Can you work these out from the model? Positions are in its coordinate system, mm. A direction names the side the tool comes from. Give positions to 0.01 mm unless a question says otherwise; leave off trailing zeros. Loops run counter-clockwise (first coordinate to the right, second up) from the corner with the lowest first, then second, coordinate; pieces in that order, holes last.
from build123d import *

# Parameters (mm, degrees)
SKETCH1_R           = 4
BOSS_EXTRUDE1_DEPTH = 5
CUT_EXTRUDE1_DEPTH  = 5


with BuildPart() as part:
    # Sketch1 → Boss-Extrude1 (new body)
    with BuildSketch(Plane.XY):
        with BuildLine():
            Line((-15, 6.5), (15, 6.5))
            ThreePointArc((15, 6.5), (21.5, 0), (15, -6.5))
            Line((15, -6.5), (-15, -6.5))
            ThreePointArc((-15, -6.5), (-21.5, 0), (-15, 6.5))
        make_face()
        with Locations((-15, 0)):
            Circle(SKETCH1_R, mode=Mode.SUBTRACT)
        with Locations((15, 0)):
            Circle(SKETCH1_R, mode=Mode.SUBTRACT)
    extrude(amount=BOSS_EXTRUDE1_DEPTH)

    # Sketch2 → Cut-Extrude1 (cut)
    with BuildSketch(Plane(origin=(21.5, 0, 0), x_dir=(0, 0, -1), z_dir=(1, 0, 0))):
        with BuildLine():
            ThreePointArc((-3.75, 0), (-2.5, -1.25), (-1.25, 0))
            Line((-1.25, 0), (-3.75, 0))
        make_face()
        with BuildLine():
            Line((-3.75, 0), (-1.25, 0))
            ThreePointArc((-1.25, 0), (-2.5, 1.25), (-3.75, 0))
        make_face()
    cut_extrude1 = extrude(amount=-CUT_EXTRUDE1_DEPTH, mode=Mode.SUBTRACT)

    # Mirror1: Cut-Extrude1 across plane
    add(cut_extrude1.mirror(Plane(origin=(0, 0, 0), x_dir=(0, 0, 1), z_dir=(1, 0, 0))), mode=Mode.SUBTRACT)


solid = part.part
(1) Suppose I cut it at A-A on y = 0. List the corners of the cut face in (x, z) for me, plus the area to 4 significant figures.
Returned:
outline: (-21.5, 0) - (-19, 0) - (-19, 1.25) - (-21.5, 1.25) - close; (-21.5, 3.75) - (-19, 3.75) - (-19, 5) - (-21.5, 5) - close; (-11, 0) - (11, 0) - (11, 5) - (-11, 5) - close; (19, 0) - (21.5, 0) - (21.5, 1.25) - (19, 1.25) - close; (19, 3.75) - (21.5, 3.75) - (21.5, 5) - (19, 5) - close
area: 122.5 mm2
(2) Which directions (+Z, -Z, +X, -X, +Y, -Y) give clear straight access to the entire face, cutting with the end or side of a thin tool? Please do faces 4 (the cylindrical face through (20.17, 0.05, 3.75)), 5 (the cylindrical face through (-20.17, 0.05, 3.75)), 6 (the flat face through (0, 0, 5)).
Returned:
face 4: +X
face 5: -X
face 6: +Z, +X, -X, +Y, -Y
(3) Suppose I cut it at C-C on x = -14.5. List the corners of the cut face in (y, z) for me.
Returned:
outline: (-6.5, 0) - (-3.97, 0) - (-3.97, 5) - (-6.5, 5) - close; (3.97, 0) - (6.5, 0) - (6.5, 5) - (3.97, 5) - close
(4) Suppose I cut it at B-B on z = 0.75. List the corners of the cut face in (x, y) for me, plus the area to 3 significant figures.
Returned:
outline: (-15, -6.5) - (15, -6.5) arc R6.5 ccw to (15, 6.5) - (-15, 6.5) arc R6.5 ccw to start; hole circle Ø8 at (-15, 0); hole circle Ø8 at (15, 0)
area: 422 mm2
(5) Please list where these lines run through material, in increasing order: probe 1 along Y at (x, z) = (15, 2.45); probe 2 along X at (y, z) = (2, 2.5); probe 3 along X at (y, z) = (1.75, 4.3).
Returned:
probe 1: y = -6.5 to -4, 4 to 6.5
probe 2: x = -21.18 to -18.46, -11.54 to 11.54, 18.46 to 21.18
probe 3: x = -21.26 to -18.6, -11.4 to 11.4, 18.6 to 21.26
(6) Will this pin go through, and if not, where does the flat tip stop? P1, Ø2, axis at y = 0, z = 2.5, coming from the +X side.
Returned:
P1: stops at x = 11.13
(7) Thinking about a two-plate mould opening in Y: for faces 1 (the cylindrical face through (11, 0, 2)), 2 (the flat face through (0, 0, 0)), 3 (the cylindrical face through (-21.5, -0.1, 0.8)), which applies, pulls with the +Y half, pulls with the -Y half, needs draft (parallel to the pull), parting line crosses it, or undercut?
Returned:
face 1: undercut
face 2: needs draft
face 3: parting line crosses it
(8) Suppose I cut it at D-D on y = 3. List the corners of the cut face in (x, z) for me, plus the area to 3 significant figures.
Returned:
outline: (-20.77, 0) - (-17.65, 0) - (-17.65, 5) - (-20.77, 5) - close; (-12.35, 0) - (12.35, 0) - (12.35, 5) - (-12.35, 5) - close; (17.65, 0) - (20.77, 0) - (20.77, 5) - (17.65, 5) - close
area: 155 mm2
